Source: CAD feature listing. Evaluate the final solid. Frame: model axes, mm. A direction names the side the tool comes from. Round coordinates to 2 decimals unless told otherwise and drop trailing zeros. Loops run counter-clockwise (first coordinate to the right, second up) from the corner with the lowest first, then second, coordinate; pieces in that order, holes last.
(1) Mould query, pull axis Y, two halves, no side actions, for faces 4 (the cylindrical face through (13.887, -10.648, 6.162)), 5 (the flat face through (0, -18, 5)), 6 (the cylindrical face through (10.382, 19.961, 7.395)), 7 (the flat face through (-0.1, 10.2, 25)). Classes: pulls with the +Y half, pulls with the -Y half, needs draft (parallel to the pull), parting line crosses it, or undercut.
(2) Section C-C, the plane y = 0. Count the separate pieces of the cut face and the enclosed holes in it, plus the area to 3 significant figures.
(3) First-contact query: pin 1 Ø8 at (y, z) = (-12.5, 4) entering from +X; pin 2 Ø4 at (y, z) = (-15.5, 18) entering from +X; pin 3 Ø0.6 at (x, y) = (0.5, -19) entering from -Z; pin 4 Ø1.8 at (x, y) = (-19.5, 0) entering from -Z. Flat tips, straight axial feed; report the tip coordinate or a pass-through.
(4) Section D-D, the plane z = 23.25. Return the cut outline in (x, y).
(5) Set-up query: faces 1 (the cylindrical face through (-4.88, 1.08, 17.32)), 2 (the flat face through (0, -19.5, 2)), 3 (the cylindrical face through (17.898, 1.021, 10.899)). Return all of +Z, -Z, +X, -X, +Y, -Y with unobstructed straight access to the full face (end or side cutting, diameter ignored); none if empty.
(6) Material intervals for probe 1 along X at (y, z) = (0, 17); probe 2 along Y at (x, z) = (0, 23.95); probe 3 along Y at (x, z) = (0, 2.75), sorted ascending.
(7) Section B-B, the plane z = 2.25. Return the cut outline in (x, y).
(8) Section A-A, the plane x = 0. Return the cut outline in (y, z), plus the area to 4 significant figures.
Solid Edge part; units mm, degrees
sketch "Sketch1" plane through (0, 0, 0) normal (0, 0, 1) x (1, 0, 0)
  circle A0 centre (0, 0) radius 22.5
extrude "Protrusion1" add sketch "Sketch1" along normal blind 20
sketch "Sketch2" plane through (0, 0, 20) normal (0, 0, 1) x (1, 0, 0)
  circle A0 centre (0, 0) radius 12.5
extrude "ProtrusioneEstrusa_2" add sketch "Sketch2" along normal blind 5
sketch "Sketch3" plane through (0, 0, 25) normal (0, 0, 1) x (1, 0, 0)
  circle A0 centre (0, 0) radius 10
extrude "ScavoEstrusione_1" cut sketch "Sketch3" against normal blind 3
chamfer "Smusso_1" distance 5 angle 45 1 edges at (-22.5, 0, 20)
sketch "Sketch4" plane through (0, 0, 22) normal (0, 0, 1) x (0, -1, 0)
  circle A0 centre (0, 0) radius 5
extrude "Cutout1" cut sketch "Sketch4" against normal through all
sketch "Sketch5" plane through (0, 0, 0) normal (0, 0, -1) x (-1, 0, 0)
  circle A0 centre (0, 0) radius 17.5
extrude "Scavo_Bobine" cut sketch "Sketch5" against normal blind 12.5
sketch "Sketch6" plane through (0, 0, 0) normal (0, 0, -1) x (0, -1, 0)
  line L0 (-14.5, -1.5) -> (-19.5, -1.5)
  line L1 (-19.5, -1.5) -> (-19.5, 1.5)
  line L2 (-19.5, 1.5) -> (-14.5, 1.5)
  line L3 (-14.5, 1.5) -> (-14.5, -1.5)
  dimension "D1" = 19.5
  dimension "D2" = 19.5
extrude "ScavoEstrusione_5" cut sketch "Sketch6" against normal blind 5
mirror "Mirror1" about plane through (0, 0, 0) normal (0, -1, 0) of "ScavoEstrusione_5"
sketch "Sketch7" plane through (0, 0, 25) normal (0, 0, 1) x (1, 0, 0)
  circle A0 centre (-19.5, 0) radius 1
extrude "Cutout2" cut sketch "Sketch7" against normal through all
sketch "Sketch8" plane through (0, 0, 25) normal (0, 0, 1) x (0, -1, 0)
  circle A0 centre (0, -19.5) radius 1.9
extrude "Scavo_Alloggio_vite" cut sketch "Sketch8" against normal blind 20
sketch "Sketch9" plane through (0, 0, 25) normal (0, 0, 1) x (0, 1, 0)
  circle A0 centre (0, -19.5) radius 1
extrude "Cutout3" cut sketch "Sketch9" against normal through all
sketch "Sketch10" plane through (0, 0, 25) normal (0, 0, 1) x (0, 1, 0)
  circle A0 centre (0, -19.5) radius 1.9
extrude "Scavo_Alloggio_vite_2" cut sketch "Sketch10" against normal blind 20
Output values:
1. face 4: undercut
1. face 5: undercut
1. face 6: parting line crosses it
1. face 7: needs draft
2. separate pieces: 4
2. enclosed holes: 0
2. area: 289 mm2
3. pin 1: stops at x = 20.83
3. pin 2: stops at x = 15.52
3. pin 3: stops at z = 5
3. pin 4: passes through
4. outline: circle Ø25 at (0, 0); hole circle Ø20 at (0, 0)
5. face 1: +Z, -Z
5. face 2: -Z
5. face 3: +Z
6. probe 1: x = -17.6 to -5, 5 to 17.6
6. probe 2: y = -12.5 to -10, 10 to 12.5
6. probe 3: y = -22.5 to -19.5, 19.5 to 22.5
7. outline: circle Ø45 at (0, 0); hole circle Ø2 at (-19.5, 0); hole (-1.5, -19.5) - (1.5, -19.5) - (1.5, -17.44) arc R17.5 ccw to (1.5, 17.44) - (1.5, 19.5) - (-1.5, 19.5) - (-1.5, 17.44) arc R17.5 ccw to (-1.5, -17.44) - close; hole circle Ø2 at (19.5, 0)
8. outline: (-22.5, 0) - (-19.5, 0) - (-19.5, 5) - (-17.5, 5) - (-17.5, 12.5) - (-5, 12.5) - (-5, 22) - (-10, 22) - (-10, 25) - (-12.5, 25) - (-12.5, 20) - (-17.5, 20) - (-22.5, 15) - close; (5, 12.5) - (17.5, 12.5) - (17.5, 5) - (19.5, 5) - (19.5, 0) - (22.5, 0) - (22.5, 15) - (17.5, 20) - (12.5, 20) - (12.5, 25) - (10, 25) - (10, 22) - (5, 22) - close
8. area: 387.5 mm2
